from build123d import *

# Parameters (mm, degrees)
SKETCH_W        = 88.55
SKETCH_H        = 51.72
PAD_DEPTH       = 15
SKETCH001_W     = 84.55
SKETCH001_H     = 47.72
POCKET_DEPTH    = 13.5
PAD001_DEPTH    = 2.5
PAD002_DEPTH    = 2.5
PAD003_DEPTH    = 2.5
PAD004_DEPTH    = 2.5
SKETCH006_R     = 1.65
HOLE_DEPTH      = 25
SKETCH007_R     = 1.65
HOLE001_DEPTH   = 25
SKETCH008_R     = 1.65
HOLE002_DEPTH   = 25
SKETCH009_R     = 1.65
HOLE003_DEPTH   = 25
SKETCH010_W     = 7
SKETCH010_H     = 19.4
POCKET001_DEPTH = 2
SKETCH011_W     = 10.5
SKETCH011_H     = 19.4
POCKET002_DEPTH = 2
SKETCH012_W     = 7.5
SKETCH012_H     = 19.4
POCKET003_DEPTH = 2
FILLET_R        = 2.5
FILLET001_R     = 2.5
FILLET002_R     = 2.5
FILLET003_R     = 2.5
FILLET004_R     = 0.5
FILLET005_R     = 0.5
FILLET006_R     = 0.5
FILLET007_R     = 0.5
PAD005_DEPTH    = 1.6
PAD006_DEPTH    = 1.6
PAD007_DEPTH    = 1.6
SKETCH016_W     = 0.7
SKETCH016_H     = 9
PAD008_DEPTH    = 1.6
SKETCH017_W     = 11.81
SKETCH017_H     = 11.81
POCKET004_DEPTH = 9.4
SKETCH018_W     = 11.81
SKETCH018_H     = 11.81
POCKET005_DEPTH = 9.4


with BuildPart() as part:
    # Sketch → Pad (new body)
    with BuildSketch(Plane.XY):
        with Locations((44.275, 25.86)):
            Rectangle(SKETCH_W, SKETCH_H)
    extrude(amount=PAD_DEPTH)

    # Sketch001 (on Face6 of Pad) → Pocket (cut)
    with BuildSketch(Plane.XY.offset(15)):
        with Locations((44.275, 25.86)):
            Rectangle(SKETCH001_W, SKETCH001_H)
    extrude(amount=-POCKET_DEPTH, mode=Mode.SUBTRACT)

    # Sketch002 (on Face11 of Pocket) → Pad001 (join)
    with BuildSketch(Plane.XY.offset(1.5)):
        with BuildLine():
            ThreePointArc((11.31, 6.81), (9.991981, 9.991981), (6.81, 11.31))
            Line((2, 11.31), (6.81, 11.31))
            Line((2, 11.31), (2, 2))
            Line((2, 2), (11.31, 2))
            Line((11.31, 6.81), (11.31, 2))
        make_face()
    extrude(amount=PAD001_DEPTH)

    # Sketch003 (on Face11 of Pad001) → Pad002 (join)
    with BuildSketch(Plane.XY.offset(1.5)):
        with BuildLine():
            ThreePointArc((6.81, 40.41), (9.991981, 41.728019), (11.31, 44.91))
            Line((11.31, 44.91), (11.31, 49.72))
            Line((2, 49.72), (11.31, 49.72))
            Line((2, 49.72), (2, 40.41))
            Line((2, 40.41), (6.81, 40.41))
        make_face()
    extrude(amount=PAD002_DEPTH)

    # Sketch004 (on Face11 of Pad002) → Pad003 (join)
    with BuildSketch(Plane.XY.offset(1.5)):
        with BuildLine():
            ThreePointArc((81.739971, 40.52), (77.24, 36.019985), (81.74, 31.52))
            Line((81.74, 31.52), (86.55, 31.52))
            Line((86.55, 31.52), (86.55, 40.52))
            Line((81.739971, 40.52), (86.55, 40.52))
        make_face()
    extrude(amount=PAD003_DEPTH)

    # Sketch005 (on Face11 of Pad003) → Pad004 (join)
    with BuildSketch(Plane.XY.offset(1.5)):
        with BuildLine():
            ThreePointArc((81.74, 11.31), (78.558019, 9.991981), (77.24, 6.81))
            Line((77.24, 6.81), (77.24, 2))
            Line((77.24, 2), (86.55, 2))
            Line((86.55, 2), (86.55, 11.31))
            Line((81.74, 11.31), (86.55, 11.31))
        make_face()
    extrude(amount=PAD004_DEPTH)

    # Sketch006 (on Face20 of Pad004) → Hole (cut)
    with BuildSketch(Plane.XY.offset(4)):
        with Locations((6.81, 44.91)):
            Circle(SKETCH006_R)
    extrude(amount=-HOLE_DEPTH, mode=Mode.SUBTRACT)

    # Sketch007 (on Face19 of Hole) → Hole001 (cut)
    with BuildSketch(Plane.XY.offset(4)):
        with Locations((6.81, 6.81)):
            Circle(SKETCH007_R)
    extrude(amount=-HOLE001_DEPTH, mode=Mode.SUBTRACT)

    # Sketch008 (on Face15 of Hole001) → Hole002 (cut)
    with BuildSketch(Plane.XY.offset(4)):
        with Locations((81.74, 6.81)):
            Circle(SKETCH008_R)
    extrude(amount=-HOLE002_DEPTH, mode=Mode.SUBTRACT)

    # Sketch009 (on Face21 of Hole002) → Hole003 (cut)
    with BuildSketch(Plane.XY.offset(4)):
        with Locations((81.74, 36.02)):
            Circle(SKETCH009_R)
    extrude(amount=-HOLE003_DEPTH, mode=Mode.SUBTRACT)

    # Sketch010 (on Face3 of Hole003) → Pocket001 (cut)
    with BuildSketch(Plane.YZ.offset(88.55)):
        with Locations((23, 15.3)):
            Rectangle(SKETCH010_W, SKETCH010_H)
    extrude(amount=-POCKET001_DEPTH, mode=Mode.SUBTRACT)

    # Sketch011 (on Face2 of Pocket001) → Pocket002 (cut)
    with BuildSketch(Plane(origin=(0, 0, 0), x_dir=(0, -1, 0), z_dir=(-1, 0, 0))):
        with Locations((-16.125, 15.3)):
            Rectangle(SKETCH011_W, SKETCH011_H)
    extrude(amount=-POCKET002_DEPTH, mode=Mode.SUBTRACT)

    # Sketch012 (on Face1 of Pocket002) → Pocket003 (cut)
    with BuildSketch(Plane.XZ):
        with Locations((64.45, 15.3)):
            Rectangle(SKETCH012_W, SKETCH012_H)
    extrude(amount=-POCKET003_DEPTH, mode=Mode.SUBTRACT)

    # Fillet
    fillet_edges = [part.edges().sort_by_distance(p)[0] for p in [
        (88.55, 0, 7.5),
    ]]
    fillet(fillet_edges, radius=FILLET_R)

    # Fillet001
    fillet001_edges = [part.edges().sort_by_distance(p)[0] for p in [
        (88.55, 51.72, 7.5),
    ]]
    fillet(fillet001_edges, radius=FILLET001_R)

    # Fillet002
    fillet002_edges = [part.edges().sort_by_distance(p)[0] for p in [
        (0, 51.72, 7.5),
    ]]
    fillet(fillet002_edges, radius=FILLET002_R)

    # Fillet003
    fillet003_edges = [part.edges().sort_by_distance(p)[0] for p in [
        (0, 0, 7.5),
    ]]
    fillet(fillet003_edges, radius=FILLET003_R)

    # Fillet004
    fillet004_edges = [part.edges().sort_by_distance(p)[0] for p in [
        (86.55, 49.72, 8.25),
    ]]
    fillet(fillet004_edges, radius=FILLET004_R)

    # Fillet005
    fillet005_edges = [part.edges().sort_by_distance(p)[0] for p in [
        (86.55, 2, 9.5),
    ]]
    fillet(fillet005_edges, radius=FILLET005_R)

    # Fillet006
    fillet006_edges = [part.edges().sort_by_distance(p)[0] for p in [
        (2, 2, 9.5),
    ]]
    fillet(fillet006_edges, radius=FILLET006_R)

    # Fillet007
    fillet007_edges = [part.edges().sort_by_distance(p)[0] for p in [
        (2, 49.72, 9.5),
    ]]
    fillet(fillet007_edges, radius=FILLET007_R)

    # Sketch013 (on Face13 of Fillet007) → Pad005 (join)
    with BuildSketch(Plane.XY.offset(4)):
        Polygon((2.7, 11.31), (2.7, 2.7), (11.31, 2.7), (11.31, 2), (2, 2), (2, 11.31), align=None)
    extrude(amount=PAD005_DEPTH)

    # Sketch014 (on Face9 of Pad005) → Pad006 (join)
    with BuildSketch(Plane.XY.offset(4)):
        Polygon((2.7, 40.41), (2.7, 49.02), (11.31, 49.02), (11.31, 49.72), (2, 49.72), (2, 40.41), align=None)
    extrude(amount=PAD006_DEPTH)

    # Sketch015 (on Face43 of Pad006) → Pad007 (join)
    with BuildSketch(Plane.XY.offset(4)):
        Polygon((85.85, 11.31), (85.85, 2.7), (77.24, 2.7), (77.24, 2), (86.55, 2), (86.55, 11.31), align=None)
    extrude(amount=PAD007_DEPTH)

    # Sketch016 (on Face43 of Pad007) → Pad008 (join)
    with BuildSketch(Plane.XY.offset(4)):
        with Locations((86.2, 36.02)):
            Rectangle(SKETCH016_W, SKETCH016_H)
    extrude(amount=PAD008_DEPTH)

    # Sketch017 (on Face2 of Pad008) → Pocket004 (cut)
    with BuildSketch(Plane.XY.offset(15)):
        with Locations((5.905, 45.815)):
            Rectangle(SKETCH017_W, SKETCH017_H)
    extrude(amount=-POCKET004_DEPTH, mode=Mode.SUBTRACT)

    # Sketch018 (on Face46 of Pocket004) → Pocket005 (cut)
    with BuildSketch(Plane.XY.offset(15)):
        with Locations((82.645, 5.905)):
            Rectangle(SKETCH018_W, SKETCH018_H)
    extrude(amount=-POCKET005_DEPTH, mode=Mode.SUBTRACT)


solid = part.part
The listing builds one solid part. Answer for the finished solid, in the listing's coordinates (mm). A direction names the side the tool comes from. Round coordinates to 2 decimals unless told otherwise and drop trailing zeros. Write each loop counter-clockwise with the first axis right and the second up, starting at its lowest first coordinate (ties: lowest second). Pieces come first, ordered by that corner, then holes. Notation, with made-up numbers: M -9,78 L 13,78 A23 cw 13,117 Z; hole C 5,12 d2. An arc over 180 degrees is marked long. Write each question's results on one line, items separated by ' | '. Start each with the question number.
Item 1: A cutting plane is placed at B-B on z = 12.25. Write down the section's boundary in (x, y) (3 decimals).
Item 2: Flat-ended cylindrical pins translate along their axes: pin 1 Ø1 at (x, z) = (88, 9.5) entering from -Y; pin 2 Ø2 at (x, y) = (87.5, 23.5) entering from +Z; pin 3 Ø4 at (x, y) = (25, 7.5) entering from -Z; pin 4 Ø3 at (y, z) = (7.5, 10) entering from +X. Find the tip coordinate at first contact, or state that the pin passes through.
Item 3: Straight lines are drawn through the part: L1, parallel to Y at x = 6.81, z = 2.9; L2, parallel to Y at x = 30.5, z = 12.75; L3, parallel to X at y = 30.5, z = 7.25. For each, find the intervals that lie inside material, in ascending order. Write a range as [from, to].
Item 4: A cutting plane is placed at D-D on z = 2.5. State how many separate pieces and enclosed holes the cut face has, and give its area (3 significant figures).
Item 5: For faces 1 (the face through (88, 23, 5.6)), 2 (the face through (83.4, 35.1, 4)), 3 (the face through (88, 19.5, 10)), 4 (the face through (11.81, 51, 10)), determine the directions among +Z, -Z, +X, -X, +Y, -Y from which every point of the face is accessible in a straight line to the end or side of a thin tool.
Item 6: For a pull along X with two mould halves and no side action, classify faces 5 (the face through (48, 49.72, 8)), 6 (the face through (77.24, 4, 3)), 7 (the face through (44, 26, 0)), 8 (the face through (0.752, 51.007, 2.839)) as pulls with the +X half, pulls with the -X half, needs draft (parallel to the pull), parting line crosses it, or undercut.
Item 7: A cutting plane is placed at C-C on x = 32. Write down the section's boundary in (y, z), and give its area (3 significant figures).
Item 8: A cutting plane is placed at A-A on y = 36.02. Write down the section's boundary in (x, z).
Check sheet entries:
1) outline: M 0,2.5 A2.5 ccw 2.5,0 L 60.7,0 L 60.7,2 L 2.5,2 A0.5 cw 2,2.5 L 2,10.875 L 0,10.875 Z; M 0,21.375 L 2,21.375 L 2,39.91 L 0,39.91 Z; M 11.81,49.72 L 86.05,49.72 A0.5 cw 86.55,49.22 L 86.55,26.5 L 88.55,26.5 L 88.55,49.22 A2.5 ccw 86.05,51.72 L 11.81,51.72 Z; M 68.2,0 L 76.74,0 L 76.74,2 L 68.2,2 Z; M 86.55,11.81 L 88.55,11.81 L 88.55,19.5 L 86.55,19.5 Z
2) pin 1: y = 11.81 | pin 2: z = 5.6 | pin 3: z = 0 | pin 4: x = 2
3) L1: [0, 5.16], [8.46, 11.31], [40.41, 43.26], [46.56, 51.72] | L2: [0, 2], [49.72, 51.72] | L3: [0, 2], [86.55, 88.55]
4) separate pieces: 1 | enclosed holes: 5 | area: 828 mm²
5) face 1: +Z, +X | face 2: +Z | face 3: +Z, +X, -X | face 4: +Z, -X, +Y
6) face 5: undercut | face 6: undercut | face 7: needs draft | face 8: pulls with the -X half
7) outline: M 0,0 L 51.72,0 L 51.72,15 L 49.72,15 L 49.72,1.5 L 2,1.5 L 2,15 L 0,15 Z | area: 132 mm²
8) outline: M 0,0 L 80.09,0 L 80.09,4 L 77.24,4 L 77.24,1.5 L 2,1.5 L 2,15 L 0,15 Z; M 83.39,0 L 88.55,0 L 88.55,15 L 86.55,15 L 86.55,5.6 L 85.85,5.6 L 85.85,4 L 83.39,4 Z
